Work out the finished part from the listing and answer in its coordinate system (mm). Coordinates: 2 decimals unless noted, no trailing zeros. Order: outer loops, then holes, each group sorted by start corner. A loop starts at its lowest first (then second) coordinate and runs counter-clockwise, first axis right, second up.
1. The part is cut by section A-A, the plane x = 0. Give the vertices of the cut face in (y, z), then the cut area to 3 significant figures.
2. The part is cut by section C-C, the plane z = -8. Give the vertices of the cut face in (x, y), then the cut area to 3 significant figures.
3. The part is cut by section B-B, the plane y = 5.5. Give the vertices of the cut face in (x, z), then the cut area to 3 significant figures.
4. Determine the mould class of faces 1 (the flat face through (0, 0, -4)), 2 (the flat face through (0, 10, -21.5)), 3 (the cylindrical face through (-20.38, 10.83, 12.63)) for opening direction Y: +Y half, -Y half, draft (parallel to the pull), parting line (faces both ways), or undercut.
5. The part is cut by section D-D, the plane y = 12. Count the separate pieces of the cut face and the enclosed holes in it, then the cut area to 3 significant figures.
6. Find the intervals of material crossed by probe 1 along X at (y, z) = (10, -16.5); probe 2 along X at (y, z) = (10, 1); probe 3 along Z at (x, y) = (-23, 18), in increasing order.
```python
from build123d import *

# Parameters (mm, degrees)
F0_W     = 60
F0_H     = 43
F0_R     = 6
F1_DEPTH = 20
F2_R     = 2.75
F3_DEPTH = 43.001
F4_R     = 2.75
F5_DEPTH = 20.001


with BuildPart() as f1:
    # F0 (on Front) → F1 (new body)
    with BuildSketch(Plane.XZ):
        Rectangle(F0_W, F0_H)
        with Locations((0, 3.5)):
            Circle(F0_R, mode=Mode.SUBTRACT)
    extrude(amount=-F1_DEPTH)

    # F2 (on face) → F3 (cut, through all)
    with BuildSketch(Plane.XY.offset(21.5)):
        with Locations((-23, 10)):
            Circle(F2_R)
        with Locations((23, 10)):
            Circle(F2_R)
    extrude(amount=-F3_DEPTH, mode=Mode.SUBTRACT)

    # F4 (on face) → F5 (cut, through all)
    with BuildSketch(Plane.XZ):
        with Locations((23, 3.5)):
            Circle(F4_R)
        with Locations((-23, -14.5)):
            Circle(F4_R)
        with Locations((23, -14.5)):
            Circle(F4_R)
        with Locations((-23, 3.5)):
            Circle(F4_R)
    extrude(amount=-F5_DEPTH, mode=Mode.SUBTRACT)


solid = f1.part
```
Geometry says:
1. outline: (0, -21.5) - (20, -21.5) - (20, -2.5) - (0, -2.5) - close; (0, 9.5) - (20, 9.5) - (20, 21.5) - (0, 21.5) - close
1. area: 620 mm2
2. outline: (-30, 0) - (30, 0) - (30, 20) - (-30, 20) - close; hole circle Ø5.5 at (-23, 10); hole circle Ø5.5 at (23, 10)
2. area: 1,150 mm2
3. outline: (-30, -21.5) - (30, -21.5) - (30, 21.5) - (-30, 21.5) - close; hole circle Ø5.5 at (-23, -14.5); hole circle Ø5.5 at (-23, 3.5); hole circle Ø12 at (0, 3.5); hole circle Ø5.5 at (23, -14.5); hole circle Ø5.5 at (23, 3.5)
3. area: 2,370 mm2
4. face 1: -Y half
4. face 2: draft
4. face 3: undercut
5. separate pieces: 3
5. enclosed holes: 1
5. area: 2,120 mm2
6. probe 1: x = -30 to -25.75, -20.25 to 20.25, 25.75 to 30
6. probe 2: x = -30 to -25.75, -20.25 to -5.45, 5.45 to 20.25, 25.75 to 30
6. probe 3: z = -21.5 to -17.25, -11.75 to 0.75, 6.25 to 21.5
